from build123d import *

# Parameters (mm, degrees)
SKETCH1_W           = 22
SKETCH1_H           = 166.3
SKETCH1_R           = 2
BOSS_EXTRUDE1_DEPTH = 5
CUT_EXTRUDE1_DEPTH  = 5
SKETCH3_W           = 22
SKETCH3_H           = 5
BOSS_EXTRUDE2_DEPTH = 6
SKETCH4_W           = 22
SKETCH4_H           = 5
CUT_EXTRUDE2_DEPTH  = 4
FILLET2_R           = 11
SKETCH5_W           = 19.280438378
SKETCH5_H           = 5
CUT_EXTRUDE3_DEPTH  = 6
SKETCH7_W           = 29.371075178
SKETCH7_H           = 5
CUT_EXTRUDE4_DEPTH  = 2


with BuildPart() as part:
    # Sketch1 → Boss-Extrude1 (new body)
    with BuildSketch(Plane(origin=(0, 0, 0), x_dir=(1, 0, 0), z_dir=(0, 1, 0))):
        with Locations((11, 83.15)):
            Rectangle(SKETCH1_W, SKETCH1_H)
        with Locations(Location((11, 5, 0), (0, 0, 270))):
            Circle(SKETCH1_R, mode=Mode.SUBTRACT)
        with Locations(Location((11, 161.3, 0), (0, 0, 270))):
            Circle(SKETCH1_R, mode=Mode.SUBTRACT)
    extrude(amount=BOSS_EXTRUDE1_DEPTH)

    # Sketch2 → Cut-Extrude1 (cut)
    with BuildSketch(Plane(origin=(0, 0, 0), x_dir=(-1, 0, 0), z_dir=(0, -1, 0))):
        with BuildLine():
            Line((-16, 30), (-16, 70))
            ThreePointArc((-16, 70), (-11, 75), (-6, 70))
            Line((-6, 70), (-6, 30))
            ThreePointArc((-6, 30), (-11, 25), (-16, 30))
        make_face()
    extrude(amount=-CUT_EXTRUDE1_DEPTH, mode=Mode.SUBTRACT)

    # Sketch3 → Boss-Extrude2 (add)
    with BuildSketch(Plane.XY):
        with Locations((11, 2.5)):
            Rectangle(SKETCH3_W, SKETCH3_H)
    extrude(amount=BOSS_EXTRUDE2_DEPTH)

    # Sketch4 → Cut-Extrude2 (cut)
    with BuildSketch(Plane.XY.offset(6)):
        with Locations((11, 2.5)):
            Rectangle(SKETCH4_W, SKETCH4_H)
    extrude(amount=-CUT_EXTRUDE2_DEPTH, mode=Mode.SUBTRACT)

    # Fillet2
    fillet2_edges = [part.edges().sort_by_distance(p)[0] for p in [
        (0, 2.5, 2),
        (22, 2.5, 2),
    ]]
    fillet(fillet2_edges, radius=FILLET2_R - 0.0001)  # a hair under: the kernel refuses the full size

    # Sketch5 → Cut-Extrude3 (cut)
    with BuildSketch(Plane.ZY):
        with Locations((-2.059665651, 2.5)):
            Rectangle(SKETCH5_W, SKETCH5_H)
    extrude(amount=-CUT_EXTRUDE3_DEPTH, mode=Mode.SUBTRACT)

    # Sketch7 → Cut-Extrude4 (cut)
    with BuildSketch(Plane(origin=(22, 0, 0), x_dir=(0, 0, -1), z_dir=(1, 0, 0))):
        with Locations((6.231522195, 2.5)):
            Rectangle(SKETCH7_W, SKETCH7_H)
    extrude(amount=-CUT_EXTRUDE4_DEPTH, mode=Mode.SUBTRACT)


solid = part.part
The model under review builds one solid part; all positions refer to its coordinate system, in mm. A direction names the side the tool comes from. Give positions to 0.01 mm unless a question says otherwise; leave off trailing zeros. Order: outer loops, then holes, each group sorted by start corner. A loop starts at its lowest first (then second) coordinate and runs counter-clockwise, first axis right, second up. Notation, with made-up numbers: M 10,24 L 51,24 A9 ccw 51,33 Z; hole C 39.5,9 d2. An arc over 180 degrees is marked long. Use one line per item in the form item = value. Start each with the question number.
Item 1: Insertion check: pin 1 Ø1 at (x, y) = (21.5, 1.5) entering from +Z. The pin has a flat end and moves straight along its axis. Give the tip position at first contact, or say it passes through.
Item 2: To check wall thickness, follow line 1 along X through (y, z) = (0.35, -68.5); line 2 along X through (y, z) = (1.4, -161.3); line 3 along Z through (x, y) = (20.5, 1.5). State the ranges of each line that lie inside material, in increasing order. Write a range as from..to.
Item 3: The part is to be moulded in two halves that separate along X. For faces 1 (the flat face through (6, 3, -6)), 2 (the flat face through (3, 2, -11.7)), 3 (the flat face through (16, 2, -50)), 4 (the cylindrical face through (16, 2.5, 0.8)), say which applies: pulls with the +X half, pulls with the -X half, needs draft (parallel to the pull), parting line crosses it, or undercut.
Item 4: We need section C-C on z = -161.3. Give the boundary of the cut face in (x, y).
Item 5: We need section B-B on y = 2.7. Give the number of separate pieces and of enclosed holes in the cut face, plus the area to 3 significant figures.
Item 6: We need section A-A on z = -5. Give the boundary of the cut face in (x, y), plus the area to 3 significant figures.
Item 7: We need section D-D on x = 2.25. Give the boundary of the cut face in (y, z), plus the area to 3 significant figures.
Item 8: For faces 5 (the cylindrical face through (11, 2, -75)), 6 (the flat face through (22, 2, -95)), 7 (the flat face through (20, 3, -12)), list the 3-axis set-ups (+Z, -Z, +X, -X, +Y, -Y) from which the entire face can be reached by the end or side of a thin tool; tool diameter is ignored.
Completed:
q1.pin_1 = -20.92
q2.line_1 = 0..6, 16..22
q2.line_2 = 0..9, 13..22
q2.line_3 = -166.3..-20.92
q3.face_1 = pulls with the -X half
q3.face_2 = needs draft
q3.face_3 = undercut
q3.face_4 = pulls with the +X half
q4.outline = M 0,0 L 9,0 L 9,5 L 0,5 Z; M 13,0 L 22,0 L 22,5 L 13,5 Z
q5.separate_pieces = 1
q5.enclosed_holes = 3
q5.area = 3,060 mm²
q6.outline = M 6,0 L 9,0 L 9,5 L 6,5 Z; M 13,0 L 20,0 L 20,5 L 13,5 Z
q6.area = 50.0 mm²
q7.outline = M 0,-166.3 L 5,-166.3 L 5,-11.7 L 0,-11.7 Z
q7.area = 773 mm²
q8.face_5 = +Y, -Y
q8.face_6 = +Z, -Z, +X, +Y, -Y
q8.face_7 = +Z, +X, +Y, -Y
